Solid Edge part; units mm, degrees
sketch "Sketch1" plane through (0, 0, 0) normal (0, 0, 1) x (1, 0, 0)
  line L0 (7.1014, 10.4369) -> (178.1014, 10.4369)
  line L1 (178.1014, 10.4369) -> (178.1014, 118.4369)
  line L2 (178.1014, 118.4369) -> (7.1014, 118.4369)
  line L3 (7.1014, 118.4369) -> (7.1014, 10.4369)
extrude "Protrusion1" add sketch "Sketch1" along normal blind 100.8
sketch "Sketch2" plane through (178.1014, 64.4369, 50.4) normal (1, 0, 0) x (0, 0, -1)
  line L0 (-50.4, -30.6) -> (32.4, 3.6)
  line L1 (32.4, 3.6) -> (32.4, 54)
  line L2 (32.4, 54) -> (-50.4, 54)
  line L3 (-50.4, 54) -> (-50.4, -30.6)
  dimension "D1" = 32.4
extrude "ExtrudedCutout_3" cut sketch "Sketch2" against normal blind 200
sketch "Sketch3" plane through (92.6014, 10.4369, 50.4) normal (0, -1, 0) x (0, 0, 1)
  line L0 (50.4, -51.3) -> (7.2, -51.3)
  line L1 (7.2, -51.3) -> (7.2, 51.3)
  line L2 (7.2, 51.3) -> (50.4, 51.3)
  line L3 (50.4, 51.3) -> (50.4, -51.3)
  dimension "D1" = 50.4
extrude "ExtrudedCutout_5" cut sketch "Sketch3" against normal blind 40
sketch "Sketch4" plane through (92.6014, 93.2369, 18) normal (0, 0, 1) x (0, 1, 0)
  line L0 (25.2, -17.1) -> (-25.2, -85.5)
  line L1 (-25.2, -85.5) -> (25.2, -85.5)
  line L2 (25.2, -85.5) -> (25.2, -17.1)
  dimension "D1" = 25.2
extrude "ExtrudedCutout_6" cut sketch "Sketch4" against normal blind 40
For this review, take the finished solid that the model builds, in its own axes (mm). A direction names the side the tool comes from. Round coordinates to 2 decimals unless told otherwise and drop trailing zeros. Order: outer loops, then holes, each group sorted by start corner. A loop starts at its lowest first (then second) coordinate and runs counter-clockwise, first axis right, second up. Notation, with made-up numbers: M 56,82 L 70,82 A8 cw 70,88 Z; hole C 74.5,-21 d7. An arc over 180 degrees is marked long. Use a Markdown table: item, result. Add a question column.
Item 1: To check wall thickness, follow line 1 along X through (y, z) = (36.5, 82.5); line 2 along Z through (x, y) = (90.5, 83.5); line 3 along Y through (x, z) = (89, 36). State the ranges of each line that lie inside material, in increasing order.
Item 2: Add section C-C, the plane z = 67. Give the boundary of the cut face in (x, y).
Item 3: Add section D-D, the plane x = 22.5. Give the boundary of the cut face in (y, z), then the cut area to 3 significant figures.
Item 4: Mouldability with a two-part tool opening along X and no side actions: class faces 4 (the flat face through (178.101, 32, 38)), 5 (the flat face through (41.301, 26, 79)), 6 (the flat face through (24, 22, 100.8)), 7 (the flat face through (143.901, 26, 80)) as released by +X, released by -X, zero draft, split by the parting line, or undercut.
Item 5: Insertion check: pin 1 (2 mm diameter, centred on x = 36, z = 35.5, fed in from +Y); pin 2 (8 mm diameter, centred on x = 66, y = 91.5, fed in from +Z); pin 3 (3.5 mm diameter, centred on x = 100, z = 59.5, fed in from -Y). Each pin has a flat end and moves straight along its axis. Give the tip position at first contact, or say it passes through.
Item 6: Add section A-A, the plane x = 61. Give the boundary of the cut face in (y, z), then the cut area to 3 significant figures.
Item 7: Tool access review of faces 1 (the flat face through (93, 30, 57.6)), 2 (the flat face through (91, 10.437, 38)), 3 (the flat face through (75, 93, 18)): name each direction out of +Z, -Z, +X, -X, +Y, -Y from which nothing blocks a thin tool from reaching the whole face with its end or side.
Item 8: Add section B-B, the plane y = 25. Give the boundary of the cut face in (x, z), then the cut area to 3 significant figures.
Geometry results:
| question | item | result |
|---|---|---|
| 1 | line 1 | x = 7.1 to 41.3, 143.9 to 178.1 |
| 1 | line 2 | z = 0 to 18 |
| 1 | line 3 | y = 10.44 to 60.6 |
| 2 | outline | M 7.1,10.44 L 41.3,10.44 L 41.3,47.8 L 7.1,47.8 Z; M 143.9,10.44 L 178.1,10.44 L 178.1,47.8 L 143.9,47.8 Z |
| 3 | outline | M 10.44,0 L 118.44,0 L 118.44,18 L 68.04,18 L 33.84,100.8 L 10.44,100.8 Z |
| 3 | area | 5,300 mm² |
| 4 | face 4 | released by +X |
| 4 | face 5 | undercut |
| 4 | face 6 | zero draft |
| 4 | face 7 | undercut |
| 5 | pin 1 | stops at y = 61.22 |
| 5 | pin 2 | stops at z = 18 |
| 5 | pin 3 | stops at y = 50.44 |
| 6 | outline | M 10.44,0 L 118.44,0 L 118.44,18 L 68.04,18 L 50.44,60.61 L 50.44,57.6 L 10.44,57.6 Z |
| 6 | area | 3,900 mm² |
| 7 | face 1 | +Z, -Y |
| 7 | face 2 | +Z, -Z, +X, -X, -Y |
| 7 | face 3 | +Z, +X, -X, +Y |
| 8 | outline | M 7.1,0 L 178.1,0 L 178.1,100.8 L 143.9,100.8 L 143.9,57.6 L 41.3,57.6 L 41.3,100.8 L 7.1,100.8 Z |
| 8 | area | 12,800 mm² |
